from build123d import *

# Parameters (mm, degrees)
SKETCH1_W           = 25.5
SKETCH1_H           = 25.4
BOSS_EXTRUDE1_DEPTH = 8.89
SKETCH2_R           = 2.5
BOSS_EXTRUDE2_DEPTH = 11.303
SKETCH3_R           = 1.25
CUT_EXTRUDE1_DEPTH  = 21.193


with BuildPart() as part:
    # Sketch1 → Boss-Extrude1 (new body)
    with BuildSketch(Plane(origin=(0, 0, 0), x_dir=(1, 0, 0), z_dir=(0, 1, 0))):
        with Locations((-4.113944862, -1.223942607)):
            Rectangle(SKETCH1_W, SKETCH1_H)
    extrude(amount=BOSS_EXTRUDE1_DEPTH)

    # Sketch2 → Boss-Extrude2 (add)
    with BuildSketch(Plane.XZ):
        with Locations((-14.577944862, 11.637942607)):
            Circle(SKETCH2_R)
        with Locations((5.919855138, 11.637942607)):
            Circle(SKETCH2_R)
        with Locations((5.919855138, -8.859857393)):
            Circle(SKETCH2_R)
        with Locations((-14.577944862, -8.859857393)):
            Circle(SKETCH2_R)
    extrude(amount=BOSS_EXTRUDE2_DEPTH)

    # Sketch3 → Cut-Extrude1 (cut, through all)
    with BuildSketch(Plane.XZ.offset(11.303)):
        with Locations((-14.577944862, 11.637942607)):
            Circle(SKETCH3_R)
        with Locations((-14.577944862, -8.859857393)):
            Circle(SKETCH3_R)
        with Locations((5.919855138, -8.859857393)):
            Circle(SKETCH3_R)
        with Locations((5.919855138, 11.637942607)):
            Circle(SKETCH3_R)
    extrude(amount=-CUT_EXTRUDE1_DEPTH, mode=Mode.SUBTRACT)


solid = part.part
Input: part model. Units: mm. Frame: model coordinates. A direction names the side the tool comes from. Coordinates: 2 decimals unless noted, no trailing zeros. Order: outer loops, then holes, each group sorted by start corner. A loop starts at its lowest first (then second) coordinate and runs counter-clockwise, first axis right, second up. Notation, with made-up numbers: M -13,-29.75 L 21,-29.75 A27 ccw 21,-11.75 Z; hole C 89,36.25 d11. An arc over 180 degrees is marked long. Answer in a Markdown table with one row per item.
(1) Section query A-A, the plane x = 6.5. Output: boundary loops of the cut face in (y, z), plus the area to 3 significant figures.
Numbers:
| item | result |
|---|---|
| outline | M -11.3,-11.29 L 0,-11.29 L 0,-11.48 L 8.89,-11.48 L 8.89,-9.97 L -11.3,-9.97 Z; M -11.3,-7.75 L 8.89,-7.75 L 8.89,10.53 L -11.3,10.53 L -11.3,9.21 L 0,9.21 L 0,-6.43 L -11.3,-6.43 Z; M -11.3,12.75 L 8.89,12.75 L 8.89,13.92 L 0,13.92 L 0,14.07 L -11.3,14.07 Z |
| area | 246 mm^2 |
(2) Contact query for flat-ended pins moving along their axis: pin 1 Ø8 at (y, z) = (-2.5, 6.5) entering from -X; pin 2 Ø12 at (x, z) = (1.5, 1) entering from -Y; pin 3 Ø2.5 at (x, y) = (-6.5, 3) entering from +Z. Output: stop coordinate, or through.
Numbers:
| item | result |
|---|---|
| pin 1 | stops at x = -16.86 |
| pin 2 | stops at y = 0 |
| pin 3 | stops at z = 13.92 |
(3) Section query D-D, the plane y = 3.5. Output: boundary loops of the cut face in (x, z).
Numbers:
| item | result |
|---|---|
| outline | M -16.86,-11.48 L 8.64,-11.48 L 8.64,13.92 L -16.86,13.92 Z; hole C -14.58,-8.86 d2.5; hole C -14.58,11.64 d2.5; hole C 5.92,-8.86 d2.5; hole C 5.92,11.64 d2.5 |
(4) Section query C-C, the plane z = 0.75. Output: boundary loops of the cut face in (x, y), plus the area to 3 significant figures.
Numbers:
| item | result |
|---|---|
| outline | M -16.86,0 L 8.64,0 L 8.64,8.89 L -16.86,8.89 Z |
| area | 227 mm^2 |
(5) Access query for faces 4 (the flat face through (5, -11.303, 13)), 5 (the cylindrical face through (7.07, -5.57, 9.42)). Directions: +Z, -Z, +X, -X, +Y, -Y. A direction counts if a zero-diameter tool reaches every point of the face in a straight line with its end or side. Return the directions, or none.
Numbers:
| item | result |
|---|---|
| face 4 | +Z, -Z, +X, -X, -Y |
| face 5 | -Y |
(6) Section query B-B, the plane y = -2.75. Output: boundary loops of the cut face in (x, z).
Numbers:
| item | result |
|---|---|
| outline | C -14.58,-8.86 d5; C -14.58,11.64 d5; C 5.92,-8.86 d5; C 5.92,11.64 d5; hole C -14.58,-8.86 d2.5; hole C -14.58,11.64 d2.5; hole C 5.92,-8.86 d2.5; hole C 5.92,11.64 d2.5 |
(7) Material intervals for line 1 (Z direction, x = 3.75, y = -10); line 2 (X direction, y = -9.75, z = -7.75); line 3 (Z direction, x = 7, y = -1.5), sorted ascending. Write a range as [from, to].
Numbers:
| item | result |
|---|---|
| line 1 | z = [-10.1, -7.62], [10.4, 12.88] |
| line 2 | x = [-16.82, -15.15], [-14, -12.34], [3.68, 5.34], [6.49, 8.16] |
| line 3 | z = [-11.11, -9.49], [-8.23, -6.61], [9.38, 11.01], [12.27, 13.89] |
(8) Draft query along Z for faces 1 (the flat face through (-4, 4, -11.476)), 2 (the cylindrical face through (5.65, -1.35, -10.08)), 3 (the flat face through (8.636, 4, 1)). Return one class per face: pulls with the +Z half, pulls with the -Z half, needs draft (parallel to the pull), parting line crosses it, or undercut.
Numbers:
| item | result |
|---|---|
| face 1 | pulls with the -Z half |
| face 2 | undercut |
| face 3 | needs draft |
